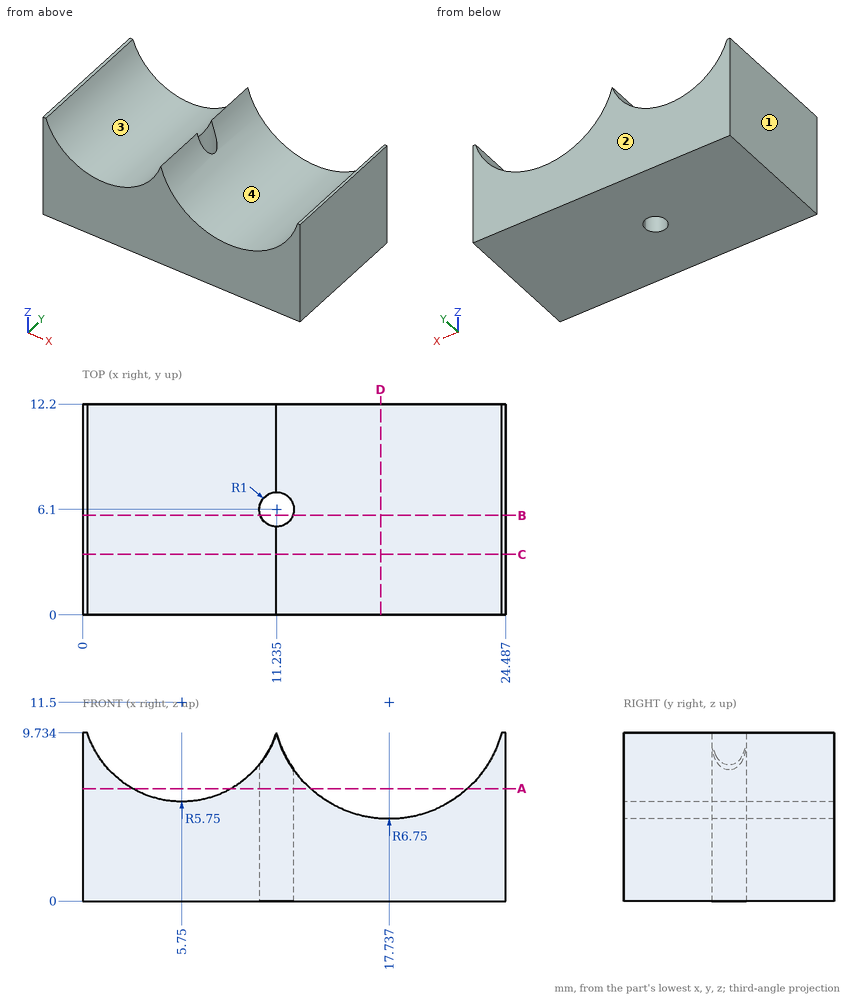
Verification items for this drawing (mm, ordinates from the low corner). Coordinates: 2 decimals unless noted, no trailing zeros. Loops run counter-clockwise (first coordinate to the right, second up) from the corner with the lowest first, then second, coordinate; pieces in that order, holes last.
Item 1: Sectioned sample at A-A, the plane z = 6.5. Record the boundary of the cut face in (x, y) (1 decimal), then the cut area to 3 significant figures.
Item 2: Sectioned sample at C-C, the plane y = 3.5. Record the boundary of the cut face in (x, z).
Item 3: Sectioned sample at B-B, the plane y = 5.75. Record the boundary of the cut face in (x, z).
Item 4: Go/stop test with flat-tipped pins: pin 1 Ø1.5 at (x, y) = (10, 6) entering from +Z (1 decimal); pin 2 Ø2 at (x, y) = (19.5, 4) entering from +Z; pin 3 Ø1.5 at (x, y) = (8, 4) entering from +Z (1 decimal). Record where each tip stops, or that it passes through.
Item 5: Release check for a two-part mould opening along X. For the marked faces 1, 2, 3 and 4 record: released by +X, released by -X, zero draft, split by the parting line, or undercut.
Item 6: Thickness scan on line 1 (X direction, y = 1.75, z = 6.75) (1 decimal); line 2 (X direction, y = 11.5, z = 8.25) (1 decimal); line 3 (Z direction, x = 15, y = 2.5). Record the ranges inside material, lowest first.
Item 7: Sectioned sample at D-D, the plane x = 17.25. Record the boundary of the cut face in (y, z).
Check result:
1. outline: (0, 0) - (2.9, 0) - (2.9, 12.2) - (0, 12.2) - close; (8.6, 0) - (13.2, 0) - (13.2, 12.2) - (8.6, 12.2) - close; (22.3, 0) - (24.5, 0) - (24.5, 12.2) - (22.3, 12.2) - close; hole (11.9, 6.9) arc R1 ccw (long way) to (12.2, 6.1) arc R1 ccw to start
1. area: 116 mm2
2. outline: (0, 0) - (24.49, 0) - (24.49, 9.73) - (24.25, 9.73) arc R6.75 cw to (11.22, 9.73) arc R5.75 cw to (0.28, 9.73) - (0, 9.73) - close
3. outline: (0, 0) - (10.3, 0) - (10.3, 7.98) arc R5.75 cw to (0.28, 9.73) - (0, 9.73) - close; (12.17, 0) - (24.49, 0) - (24.49, 9.73) - (24.25, 9.73) arc R6.75 cw to (12.17, 7.68) - close
4. pin 1: stops at z = 8.2
4. pin 2: stops at z = 5.34
4. pin 3: stops at z = 6.6
5. face 1: released by -X
5. face 2: zero draft
5. face 3: undercut
5. face 4: undercut
6. line 1: x = 0 to 2.5, 9 to 12.9, 22.5 to 24.5
6. line 2: x = 0 to 1, 10.5 to 11.8, 23.7 to 24.5
6. line 3: z = 0 to 5.33
7. outline: (0, 0) - (12.2, 0) - (12.2, 4.77) - (0, 4.77) - close
